Autodesk Inventor part; units mm, degrees
ref_plane "YZ Plane" through (0, 0, 0) normal (1, 0, 0) x (0, 1, 0)
ref_plane "XZ Plane" through (0, 0, 0) normal (0, 1, 0) x (-1, 0, 0)
ref_plane "XY Plane" through (0, 0, 0) normal (0, 0, 1) x (1, 0, 0)
sketch "Sketch1" plane through (0, 0, 0) normal (0, 0, 1) x (1, 0, 0)
  circle A0 centre (13.2036, 20.3187) radius 2.2225
  circle A1 centre (-12.1964, 20.3187) radius 2.2225
  arc A2 (17.764, 18.9458) -> (13.2036, 25.0812) centre (13.2036, 20.3187) ccw
  arc A3 (-12.1964, 25.0812) -> (-16.7567, 18.9458) centre (-12.1964, 20.3187) ccw
  line L0 (13.2036, 25.0812) -> (-12.1964, 25.0812)
  line L1 (7.3873, -15.5216) -> (17.764, 18.9458)
  line L2 (4.3471, -17.7813) -> (-3.3398, -17.7813)
  line L3 (-6.38, -15.5216) -> (-16.7567, 18.9458)
  arc A4 (4.3471, -17.7813) -> (7.3873, -15.5216) centre (4.3471, -14.6063) ccw
  arc A5 (-6.38, -15.5216) -> (-3.3398, -17.7813) centre (-3.3398, -14.6063) ccw
  point P0 (0, 0)
  point P1 (6.707, -17.7813)
  dimension "d0" = 38.1
  dimension "d1" = 3.175
  dimension "d2" = 4.7625
  dimension "d3" = 4.7625
extrude "Extrusion1" add sketch "Sketch1" along normal blind 1.5875
properties part number "hoook_gusset" material "Acetal Resin, White"
Here's how the part is built. I have some questions about the finished solid (model axes, mm). Coordinates: 2 decimals unless noted, no trailing zeros. Write each loop counter-clockwise with the first axis right and the second up, starting at its lowest first coordinate (ties: lowest second). Pieces come first, ordered by that corner, then holes. Notation, with made-up numbers: (45.5, 68) - (102.5, 68) arc R24 cw to (102.5, 99) - close; hole circle Ø10 at (29.5, 73). An arc over 180 degrees is marked (long way). Use one line per item in the form item = value.
1) Suppose I cut it at D-D, the plane x = -11. Write out the boundary of the cut face in (y, z).
Solved:
outline = (-0.18, 0) - (18.45, 0) - (18.45, 1.59) - (-0.18, 1.59) - close; (22.19, 0) - (25.08, 0) - (25.08, 1.59) - (22.19, 1.59) - close
2) Suppose I cut it at A-A, the plane x = 14. Write out the boundary of the cut face in (y, z), plus the area to 3 significant figures.
Solved:
outline = (6.44, 0) - (18.24, 0) - (18.24, 1.59) - (6.44, 1.59) - close; (22.39, 0) - (25.01, 0) - (25.01, 1.59) - (22.39, 1.59) - close
area = 22.9 mm2
3) Suppose I cut it at B-B, the plane z = 0.5. Write out the boundary of the cut face in (x, y) (1 decimal).
Solved:
outline = (-16.8, 18.9) - (-6.4, -15.5) arc R3.2 ccw to (-3.3, -17.8) - (4.3, -17.8) arc R3.2 ccw to (7.4, -15.5) - (17.8, 18.9) arc R4.8 ccw to (13.2, 25.1) - (-12.2, 25.1) arc R4.8 ccw to start; hole circle Ø4.4 at (-12.2, 20.3); hole circle Ø4.4 at (13.2, 20.3)
4) I'm going to push a flat-ended pin straight in: P1, Ø4, axis at x = -11, y = 13.5, coming from the -Z side. Where does the tip first touch, or does it pass through?
Solved:
P1 = 0
5) I need wall thicknesses on line 1 (Y direction, x = -3.5, z = 0.4); line 2 (Y direction, x = -5, z = 0.1); line 3 (X direction, y = -15, z = 1.4). Which ranges of each line are inside material? Lowest first, please.
Solved:
line_1 = -17.78 to 25.08
line_2 = -17.31 to 25.08
line_3 = -6.54 to 7.54
6) Suppose I cut it at C-C, the plane y = -10.5. Write out the boundary of the cut face in (x, z).
Solved:
outline = (-7.89, 0) - (8.9, 0) - (8.9, 1.59) - (-7.89, 1.59) - close
7) Thinking about a two-plate mould opening in X: for faces 1 (the cylindrical face through (-12.486, 18.115, 0.783)), 2 (the cylindrical face through (16.99, 23.21, 0.78)), 3 (the cylindrical face through (12.914, 18.115, 0.783)), 4 (the cylindrical face through (-16.055, 23.11, 0.783)), which applies, released by +X, released by -X, zero draft, split by the parting line, or undercut?
Solved:
face_1 = undercut
face_2 = released by +X
face_3 = undercut
face_4 = released by -X
